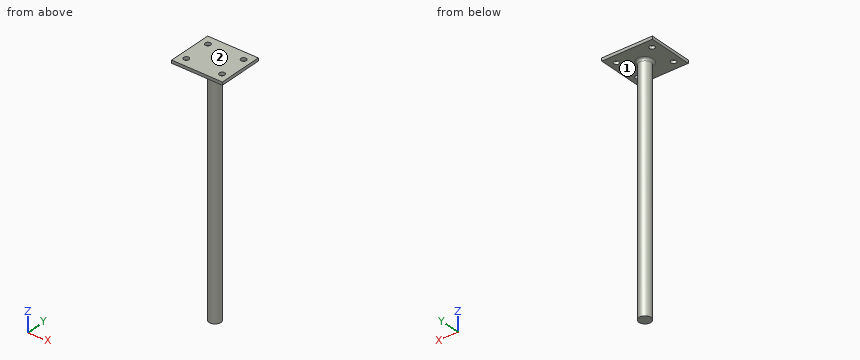
from build123d import *

# Parameters (mm, degrees)
SKETCH1_W           = 34
SKETCH1_H           = 30
SKETCH1_R           = 1.8
BOSS_EXTRUDE1_DEPTH = 2
SCALE1_SCALE        = 1.25
SKETCH2_R           = 5
BOSS_EXTRUDE3_DEPTH = 200
FILLET2_R           = 2


with BuildPart() as part:
    # Sketch1 → Boss-Extrude1 (new body)
    with BuildSketch(Plane.XY):
        Rectangle(SKETCH1_W, SKETCH1_H)
        with Locations((-12, 9)):
            Circle(SKETCH1_R, mode=Mode.SUBTRACT)
        with Locations((12, 9)):
            Circle(SKETCH1_R, mode=Mode.SUBTRACT)
        with Locations((12, -9)):
            Circle(SKETCH1_R, mode=Mode.SUBTRACT)
        with Locations((-12, -9)):
            Circle(SKETCH1_R, mode=Mode.SUBTRACT)
    extrude(amount=BOSS_EXTRUDE1_DEPTH)


with BuildPart() as part_1:
    # Scale1: scaled about (0, 0, 1)
    add(part.part.scale(SCALE1_SCALE).moved(Location((0, 0, -0.25))))

    # Sketch2 → Boss-Extrude3 (add)
    with BuildSketch(Plane(origin=(0, 0, -0.25), x_dir=(-1, 0, 0), z_dir=(0, 0, -1))):
        Circle(SKETCH2_R)
    extrude(amount=BOSS_EXTRUDE3_DEPTH)

    # Fillet2
    fillet2_edges = [part_1.edges().sort_by_distance(p)[0] for p in [
        (5, 0, -0.25),
    ]]
    fillet(fillet2_edges, radius=FILLET2_R)


solid = part_1.part
Geometry check sheet. Reference: the model listing, model coordinates, mm. Face numbers are marked on the shaded views. A direction names the side the tool comes from. Coordinates: 2 decimals unless noted, no trailing zeros. Order: outer loops, then holes, each group sorted by start corner. A loop starts at its lowest first (then second) coordinate and runs counter-clockwise, first axis right, second up. Notation, with made-up numbers: (67.25, 57.5) -> (94.25, 57.5) arc R30 cw to (94.25, 84.5) -> close; hole circle Ø9 at (1.25, 69.25). An arc over 180 degrees is marked (long way). Use a Markdown table: item, result. Add a question column.
1. Go/stop test with flat-tipped pins: pin 1 Ø7 at (x, y) = (-15, 11.25) entering from -Z; pin 2 Ø10 at (y, z) = (1, -139.5) entering from +X. Record where each tip stops, or that it passes through.
2. Material ranges on L1, parallel to Y at x = -15, z = 0; L2, parallel to Z at x = -16.5, y = -9; L3, parallel to Z at x = 6, y = 2, recorded low to high.
3. Cross-section at C-C (y = 0). Enter the section's corners in (x, z), and give its area (3 significant figures).
4. Cross-section at D-D (z = -150). Enter the section's corners in (x, y), and give its area (3 significant figures).
5. Set-up check for the marked faces 1 and 2: record each of +Z, -Z, +X, -X, +Y, -Y from which the full face is reachable in a straight line by a thin tool's end or side.
6. Cross-section at B-B (x = 15). Enter the section's corners in (y, z), and give its area (4 significant figures).
7. Cross-section at A-A (y = -11.25). Enter the section's corners in (x, z), and give its area (4 significant figures).
Filled sheet:
| question | item | result |
|---|---|---|
| 1 | pin 1 | z = -0.25 |
| 1 | pin 2 | x = 5 |
| 2 | L1 | -18.75 to -13.5, -9 to 9, 13.5 to 18.75 |
| 2 | L2 | -0.25 to 2.25 |
| 2 | L3 | -0.37 to 2.25 |
| 3 | outline | (-21.25, -0.25) -> (-7, -0.25) arc R2 cw to (-5, -2.25) -> (-5, -200.25) -> (5, -200.25) -> (5, -2.25) arc R2 cw to (7, -0.25) -> (21.25, -0.25) -> (21.25, 2.25) -> (-21.25, 2.25) -> close |
| 3 | area | 2,110 mm2 |
| 4 | outline | circle Ø10 at (0, 0) |
| 4 | area | 78.5 mm2 |
| 5 | face 1 | -Z |
| 5 | face 2 | +Z, +X, -X, +Y, -Y |
| 6 | outline | (-18.75, -0.25) -> (-13.5, -0.25) -> (-13.5, 2.25) -> (-18.75, 2.25) -> close; (-9, -0.25) -> (9, -0.25) -> (9, 2.25) -> (-9, 2.25) -> close; (13.5, -0.25) -> (18.75, -0.25) -> (18.75, 2.25) -> (13.5, 2.25) -> close |
| 6 | area | 71.25 mm2 |
| 7 | outline | (-21.25, -0.25) -> (-17.25, -0.25) -> (-17.25, 2.25) -> (-21.25, 2.25) -> close; (-12.75, -0.25) -> (12.75, -0.25) -> (12.75, 2.25) -> (-12.75, 2.25) -> close; (17.25, -0.25) -> (21.25, -0.25) -> (21.25, 2.25) -> (17.25, 2.25) -> close |
| 7 | area | 83.75 mm2 |
